Autodesk Inventor part; units mm, degrees
ref_plane "YZ Plane" through (0, 0, 0) normal (1, 0, 0) x (0, 1, 0)
ref_plane "XZ Plane" through (0, 0, 0) normal (0, 1, 0) x (-1, 0, 0)
ref_plane "XY Plane" through (0, 0, 0) normal (0, 0, 1) x (1, 0, 0)
sketch "Sketch1" plane through (0, 0, 0) normal (0, 1, 0) x (-1, 0, 0)
  line L0 (19, 96) -> (-160, 96)
  line L1 (-160, 96) -> (-160, 26)
  line L2 (-160, 26) -> (19, 26)
  line L3 (19, 26) -> (19, 96)
  point P0 (0, 0)
  dimension "d0" = 179
  dimension "d1" = 70
extrude "Extrusion1" add sketch "Sketch1" along normal blind 8
sketch "Sketch2" plane through (0, 8, 0) normal (0, 1, 0) x (1, 0, 0)
  circle A0 centre (-29, -61) radius 10
  line L0 (-29, -71) -> (-14.7125, -71)
  line L1 (-29, -51) -> (-14.2875, -51)
  line L2 (-14.7125, -71) -> (-14.2875, -51)
  line L3 (160, -26) -> (-19, -26)
  line L4 (70.5, -26) -> (70.5, -114.3)
  circle A1 centre (170, -61) radius 10
  line L5 (170, -71) -> (155.7125, -71)
  line L6 (170, -51) -> (155.2875, -51)
  line L7 (155.7125, -71) -> (155.2875, -51)
  line L8 (-19, -96) -> (160, -96)
  line L9 (-19, -26) -> (-19, -96)
  point P0 (0, 0)
  point P1 (-19, -61)
  dimension "d5" = 20
  dimension "d14" = 25
  dimension "d16" = 10
extrude "Extrusion2" add sketch "Sketch2" against normal blind 8 contours A0 | L9 L0 A0 | A0 L1 L9 | L9 L1 L2 L0 | A1 | A1 L5 L7 L6
sketch "Sketch3" plane through (0, 8, 0) normal (0, 1, 0) x (1, 0, 0)
  arc A0 (-29, -51) -> (-29, -71) centre (-29, -61) ccw
  circle A1 centre (-29, -61) radius 2.5
  arc A2 (170, -71) -> (170, -51) centre (170, -61) ccw
  circle A3 centre (170, -61) radius 2.5
  point P0 (0, 0)
  dimension "d8" = 5
  dimension "d9" = 5
extrude "Extrusion3" cut sketch "Sketch3" against normal blind 8
sketch "Sketch4" plane through (0, 8, 0) normal (0, 1, 0) x (1, 0, 0)
  line L0 (-19, -26) -> (-19, -96)
  line L1 (-19, -41.275) -> (-45.0875, -41.275)
  line L2 (-45.0875, -41.275) -> (-45.0875, -80.9625)
  line L3 (-45.0875, -80.9625) -> (-19, -80.9625)
  line L4 (-19, -80.9625) -> (-19, -41.275)
  line L5 (160, -96) -> (160, -26)
  line L6 (160, -41.275) -> (180.975, -41.275)
  line L7 (180.975, -41.275) -> (180.975, -82.55)
  line L8 (180.975, -82.55) -> (160, -82.55)
  line L9 (160, -82.55) -> (160, -41.275)
  point P0 (0, 0)
  point P1 (-19, -51)
  point P2 (160, -51)
  point P3 (160, -82.55)
  point P4 (-19, -80.9625)
extrude "Extrusion4" cut sketch "Sketch4" against normal blind 4
properties part number "Fuslage cover"
Could you check a few things on this model? Use its own coordinates, in mm. A direction names the side the tool comes from. Give positions to 0.01 mm unless a question says otherwise; leave off trailing zeros. Write each loop counter-clockwise with the first axis right and the second up, starting at its lowest first coordinate (ties: lowest second). Pieces come first, ordered by that corner, then holes. Notation, with made-up numbers: (-29, -21) -> (-18, -21) arc R9 cw to (-18, -8) -> close; hole circle Ø5 at (46, -24.75). An arc over 180 degrees is marked (long way). Answer as a JSON object with one key per item and string values.
Q1. Will these pins go through, and if not, where does the flat tip stop? pin 1 Ø22 at (x, z) = (-31, 59.5) entering from +Y; pin 2 Ø1 at (x, z) = (134.5, 70.5) entering from -Y; pin 3 Ø3 at (x, y) = (165, 1) entering from -Z; pin 4 Ø4 at (y, z) = (3.5, 65.5) entering from +X.
Taken from the geometry:
{"pin 1": "stops at y = 4", "pin 2": "stops at y = 0", "pin 3": "stops at z = 51", "pin 4": "stops at x = 179.68"}
Q2. Suppose I cut it at B-B on y = 2.75. Write out the boundary of the cut face in (x, z), then the cut area to 3 significant figures.
Taken from the geometry:
{"outline": "(-29, 51) -> (-19, 51) -> (-19, 26) -> (160, 26) -> (160, 51) -> (170, 51) arc R10 ccw to (170, 71) -> (160, 71) -> (160, 96) -> (-19, 96) -> (-19, 71) -> (-29, 71) arc R10 ccw to start; hole circle Ø5 at (-29, 61); hole circle Ø5 at (170, 61)", "area": "13,200 mm²"}
Q3. Suppose I cut it at C-C on z = 76. Write out the boundary of the cut face in (x, y).
Taken from the geometry:
{"outline": "(-19, 0) -> (160, 0) -> (160, 8) -> (-19, 8) -> close"}
Q4. We'd pull the mould along X, two halves only. Please class faces 4 (the flat face through (-24, 2, 71)), 5 (the cylindrical face through (-39, 2, 61)), 6 (the cylindrical face through (-30.84, 2.03, 59.31)): released by +X, released by -X, zero draft, split by the parting line, or undercut.
Taken from the geometry:
{"face 4": "zero draft", "face 5": "released by -X", "face 6": "undercut"}
Q5. Which directions (+Z, -Z, +X, -X, +Y, -Y) give clear straight access to the entire face, cutting with the end or side of a thin tool? Please do faces 1 (the flat face through (165, 2, 71)), 2 (the flat face through (-24, 2, 51)), 3 (the flat face through (168, 4, 63)).
Taken from the geometry:
{"face 1": "+Z, +X, +Y, -Y", "face 2": "-Z, -X, +Y, -Y", "face 3": "+Z, -Z, +X, +Y"}
Q6. Suppose I cut it at A-A on z = 61. Write out the boundary of the cut face in (x, y).
Taken from the geometry:
{"outline": "(-39, 0) -> (-31.5, 0) -> (-31.5, 4) -> (-39, 4) -> close; (-26.5, 0) -> (167.5, 0) -> (167.5, 4) -> (160, 4) -> (160, 8) -> (-19, 8) -> (-19, 4) -> (-26.5, 4) -> close; (172.5, 0) -> (180, 0) -> (180, 4) -> (172.5, 4) -> close"}
Q7. Please list where these lines run through material, in increasing order: L1, parallel to X at y = 2.65, z = 61; L2, parallel to Z at x = 170, y = 1; L3, parallel to X at y = 4.5, z = 67.5.
Taken from the geometry:
{"L1": "x = -39 to -31.5, -26.5 to 167.5, 172.5 to 180", "L2": "z = 51 to 58.5, 63.5 to 71", "L3": "x = -19 to 160"}
